Geometry: final body of the model. Coordinates: model frame, mm. A direction names the side the tool comes from. Round coordinates to 2 decimals unless told otherwise and drop trailing zeros. Loops run counter-clockwise (first coordinate to the right, second up) from the corner with the lowest first, then second, coordinate; pieces in that order, holes last. Notation, with made-up numbers: M -6,56.25 L 13,56.25 A20 cw 13,65.25 Z; hole C 85.25,36.25 d9. An arc over 180 degrees is marked long. Write each question's results on one line, items separated by ' | '.
```python
from build123d import *

# Parameters (mm, degrees)
F1_DEPTH = 450
F2_T     = -3
F3_W     = 60
F3_H     = 450
F4_DEPTH = 3
F6_DEPTH = 3
F8_DEPTH = 3


with BuildPart() as f1:
    # F0 (on Front) → F1 (new body)
    with BuildSketch(Plane.XZ):
        Polygon((330, 990), (-330, 990), (-330, 0), (0, 0), (330, 0), align=None)
    extrude(amount=F1_DEPTH)

    # F2
    f2_openings = [f1.faces().sort_by_distance(p)[0] for p in [
        (0, -450, 495),
        (0, -225, 990),
        (0, 0, 495),
    ]]
    offset(amount=F2_T, openings=f2_openings)

    # F3 (on face) → F4 (join)
    with BuildSketch(Plane.XY.offset(990)):
        with Locations((-357, -225)):
            Rectangle(F3_W, F3_H)
        with Locations((357, -225)):
            Rectangle(F3_W, F3_H)
    extrude(amount=-F4_DEPTH)

    # F5 (on face) → F6 (join)
    with BuildSketch(Plane(origin=(0, 0, 0), x_dir=(-1, 0, 0), z_dir=(0, 1, 0))):
        Polygon((387, 990), (327, 990), (327, 3), (-327, 3), (-327, 990), (-387, 990), (-387, -50), (22.530401, -50), (387, -50), align=None)
    extrude(amount=F6_DEPTH)

    # F7 (on face) → F8 (join)
    with BuildSketch(Plane.XZ.offset(450)):
        Polygon((387, -50), (387, 990), (327, 990), (327, 3), (-327, 3), (-327, 990), (-387, 990), (-387, -50), (35.580868, -50), align=None)
    extrude(amount=F8_DEPTH)


solid = f1.part
```
1. Section A-A (z = 507.5). Output: boundary loops of the cut face in (x, y), then the cut area to 3 significant figures.
Answer key:
outline: M -387,-453 L -327,-453 L -327,3 L -387,3 L -387,0 L -330,0 L -330,-450 L -387,-450 Z; M 327,-453 L 387,-453 L 387,-450 L 330,-450 L 330,0 L 387,0 L 387,3 L 327,3 Z | area: 3,420 mm²
2. Ray query, probe 1 along X at (y, z) = (-264.5, 166); probe 2 along Z at (x, y) = (308.5, -249); probe 3 along Y at (x, z) = (-347, 744.5). Return the intervals inside material, ascending.
Answer key:
probe 1: x = -330 to -327, 327 to 330 | probe 2: z = 0 to 3 | probe 3: y = -453 to -450, 0 to 3
3. Section C-C (y = -34.5). Output: boundary loops of the cut face in (x, z).
Answer key:
outline: M -387,987 L -330,987 L -330,0 L 330,0 L 330,987 L 387,987 L 387,990 L 327,990 L 327,3 L -327,3 L -327,990 L -387,990 Z
4. Section B-B (x = -241). Output: boundary loops of the cut face in (y, z).
Answer key:
outline: M -453,-50 L -450,-50 L -450,0 L 0,0 L 0,-50 L 3,-50 L 3,3 L -453,3 Z
5. Draft query along X for faces 4 (the face through (-330, -222, 500)), 5 (the face through (-327, -222, 490)), 6 (the face through (346, 3, 357)), 7 (the face through (327, -222, 503)). Return one class per face: pulls with the +X half, pulls with the -X half, needs draft (parallel to the pull), parting line crosses it, or undercut.
Answer key:
face 4: pulls with the -X half | face 5: undercut | face 6: needs draft | face 7: undercut
6. Pin query (flat end, axial travel): P1, Ø1.5, axis at x = 188, y = -164, coming from the -Z side; P2, Ø17, axis at x = 353.5, y = -250.5, coming from the -Z side; P3, Ø2, axis at x = 151, y = -158, coming from the +Z side. Return the tip coordinate at first contact, or that it passes through.
Answer key:
P1: stops at z = 0 | P2: stops at z = 987 | P3: stops at z = 3
7. Access query for faces 1 (the face through (346, 0, 356)), 2 (the face through (-359, -222, 987)), 3 (the face through (-5, -222, 0)). Directions: +Z, -Z, +X, -X, +Y, -Y. A direction counts if a zero-diameter tool reaches every point of the face in a straight line with its end or side. Return the directions, or none.
Answer key:
face 1: -Z | face 2: -Z, -X | face 3: -Z, +X, -X
